The listing builds one solid part. Answer for the finished solid, in the listing's coordinates (mm). A direction names the side the tool comes from. Give positions to 0.01 mm unless a question says otherwise; leave off trailing zeros. Loops run counter-clockwise (first coordinate to the right, second up) from the corner with the lowest first, then second, coordinate; pieces in that order, holes last. Notation, with made-up numbers: M 15.5,55 L 64.5,55 A27 cw 64.5,81 Z; hole C -33,36.25 d8. An arc over 180 degrees is marked long. Return JSON: item names as keys, results as strings.
from build123d import *

# Parameters (mm, degrees)
F0_W     = 38.1
F0_H     = 12.7
F1_DEPTH = 12.7
F3_DEPTH = 76.2
F4_DEPTH = 38.101
F5_DEPTH = 38.101


with BuildPart() as f1:
    # F0 (on Front) → F1 (new body)
    with BuildSketch(Plane.XZ):
        Polygon((0, 25.4), (0, 0), (38.1, 38.1), (76.2, 0), (76.2, 25.4), (50.8, 50.8), (25.4, 50.8), align=None)
        Polygon((38.1, 38.1), (0, 0), (19.05, 0), (19.05, 12.7), (57.15, 12.7), (57.15, 0), (76.2, 0), align=None)
        with Locations((38.1, 6.35)):
            Rectangle(F0_W, F0_H)
    extrude(amount=-F1_DEPTH)

    # F2 (on Right) → F3 (join)
    with BuildSketch(Plane.YZ):
        Polygon((-38.1, 0), (0, 0), (0, 38.1), align=None)
    extrude(amount=F3_DEPTH)

    # F4 (cut, through all): faces of the model
    f4_faces = [f1.faces().sort_by_distance(p)[0] for p in [
        (4.2333333333, 0, 33.8666666667),
        (71.9666666667, 0, 33.8666666667),
    ]]
    extrude(f4_faces, amount=-F4_DEPTH, mode=Mode.SUBTRACT)

    # F0 (on Front) → F5 (cut, through all)
    with BuildSketch(Plane.XZ):
        with Locations((38.1, 6.35)):
            Rectangle(F0_W, F0_H)
    extrude(amount=F5_DEPTH, mode=Mode.SUBTRACT)


solid = f1.part
(1) Determine the mould class of faces 3 (the flat face through (38, 0, 6)), 4 (the flat face through (38, 0, 43)), 5 (the flat face through (76.2, -7, 13)) for opening direction X: released by +X, released by -X, zero draft, split by the parting line, or undercut.
Values follow:
{"face 3": "undercut", "face 4": "zero draft", "face 5": "released by +X"}
(2) The part is cut by section A-A (x = 48). Determine the outline of the cut face in (y, z), and give its area (3 significant figures).
Values follow:
{"outline": "M -25.4,12.7 L 0,12.7 L 0,0 L 12.7,0 L 12.7,50.8 L 0,50.8 L 0,38.1 Z", "area": "968 mm²"}
(3) The part is cut by section C-C (z = 9). Determine the outline of the cut face in (x, y), and give its area (3 significant figures).
Values follow:
{"outline": "M 0,-29.1 L 19.05,-29.1 L 19.05,0 L 57.15,0 L 57.15,-29.1 L 76.2,-29.1 L 76.2,12.7 L 0,12.7 Z", "area": "2,080 mm²"}
(4) The part is cut by section B-B (y = -11.5). Determine the outline of the cut face in (x, z).
Values follow:
{"outline": "M 0,0 L 19.05,0 L 19.05,12.7 L 57.15,12.7 L 57.15,0 L 76.2,0 L 76.2,25.4 L 75,26.6 L 1.2,26.6 L 0,25.4 Z"}
(5) Given pin 1 (10 mm diameter, centred on x = 36, y = -6, fed in from -Z); pin 2 (6 mm diameter, centred on x = 30, y = -21.5, fed in from +Z); pin 3 (1 mm diameter, centred on x = 8, y = -16.5, fed in from +Z), each flat-ended and moving along its own axis, determine where each tip first touches the part or whether it passes through.
Values follow:
{"pin 1": "z = 12.7", "pin 2": "z = 19.6", "pin 3": "z = 22.1"}
(6) A tool of negligible diameter and unlimited length cuts with its end or side. For faces 1 (the flat face through (37.6, -14.5, 23.6)), 2 (the flat face through (19.05, -15, 6)), from which of +Z, -Z, +X, -X, +Y, -Y can it reach the whole face along a straight path? Write none if from no direction.
Values follow:
{"face 1": "+Z, +X, -X, -Y", "face 2": "-Z, -Y"}
(7) Straight lines are drawn through the part: line 1 along X through (y, z) = (-12, 5); line 2 along Y through (x, z) = (20, 11); line 3 along Y through (x, z) = (39.5, 17.5). For each, find the intervals that lie inside material, in ascending order.
Values follow:
{"line 1": "0 to 19.05, 57.15 to 76.2", "line 2": "0 to 12.7", "line 3": "-20.6 to 12.7"}
(8) The part is cut by section D-D (y = -1.5). Determine the outline of the cut face in (x, z), and give its area (3 significant figures).
Values follow:
{"outline": "M 0,0 L 19.05,0 L 19.05,12.7 L 57.15,12.7 L 57.15,0 L 76.2,0 L 76.2,25.4 L 65,36.6 L 11.2,36.6 L 0,25.4 Z", "area": "2,180 mm²"}
